Can you work these out from the drawing? Everything is in mm from the part's minimum corner. Round coordinates to 2 decimals unless told otherwise and drop trailing zeros. Order: outer loops, then holes, each group sorted by start corner. A loop starts at its lowest first (then second) coordinate and runs counter-clockwise, first axis right, second up. Notation, with made-up numbers: M 85,2 L 97,2 A17 cw 97,6 Z; hole C 61.5,45 d4. An arc over 180 degrees is marked long. Write each question's results on one line, items separated by ' | '. Start each with the question number.
1. Suppose I cut it at C-C on z = 0.35. Write out the boundary of the cut face in (x, y).
2. Suppose I cut it at B-B on x = 20.55. Write out the boundary of the cut face in (y, z).
3. Suppose I cut it at A-A on y = 3.36. Write out the boundary of the cut face in (x, z), and give its area (3 significant figures).
4. I'm going to push flat-ended pins straight in: pin 1 (2.5 mm diameter, centred on x = 3.5, y = 3.36, fed in from +Z); pin 2 (10 mm diameter, centred on x = 8, y = 13, fed in from -Z). Where does each tip first touch, or does it pass through?
5. Please list where these lines run through material, in increasing order: L1, parallel to Y at x = 20.55, z = 0.7; L2, parallel to Y at x = 3, z = 0.3.
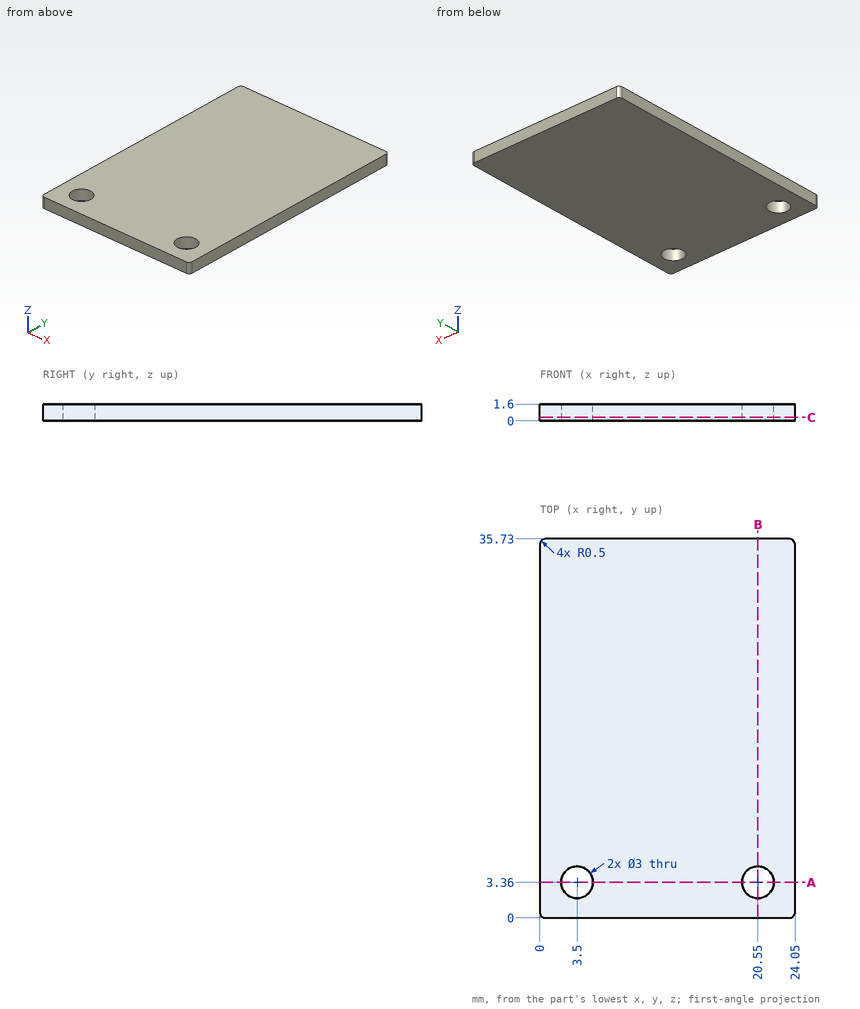
Filled sheet:
1) outline: M 0,0.5 A0.5 ccw 0.5,0 L 23.55,0 A0.5 ccw 24.05,0.5 L 24.05,35.23 A0.5 ccw 23.55,35.73 L 0.5,35.73 A0.5 ccw 0,35.23 Z; hole C 3.5,3.36 d3; hole C 20.55,3.36 d3
2) outline: M 0,0 L 1.86,0 L 1.86,1.6 L 0,1.6 Z; M 4.86,0 L 35.73,0 L 35.73,1.6 L 4.86,1.6 Z
3) outline: M 0,0 L 2,0 L 2,1.6 L 0,1.6 Z; M 5,0 L 19.05,0 L 19.05,1.6 L 5,1.6 Z; M 22.05,0 L 24.05,0 L 24.05,1.6 L 22.05,1.6 Z | area: 28.9 mm^2
4) pin 1: passes through | pin 2: stops at z = 0
5) L1: y = 0 to 1.86, 4.86 to 35.73 | L2: y = 0 to 1.95, 4.77 to 35.73
